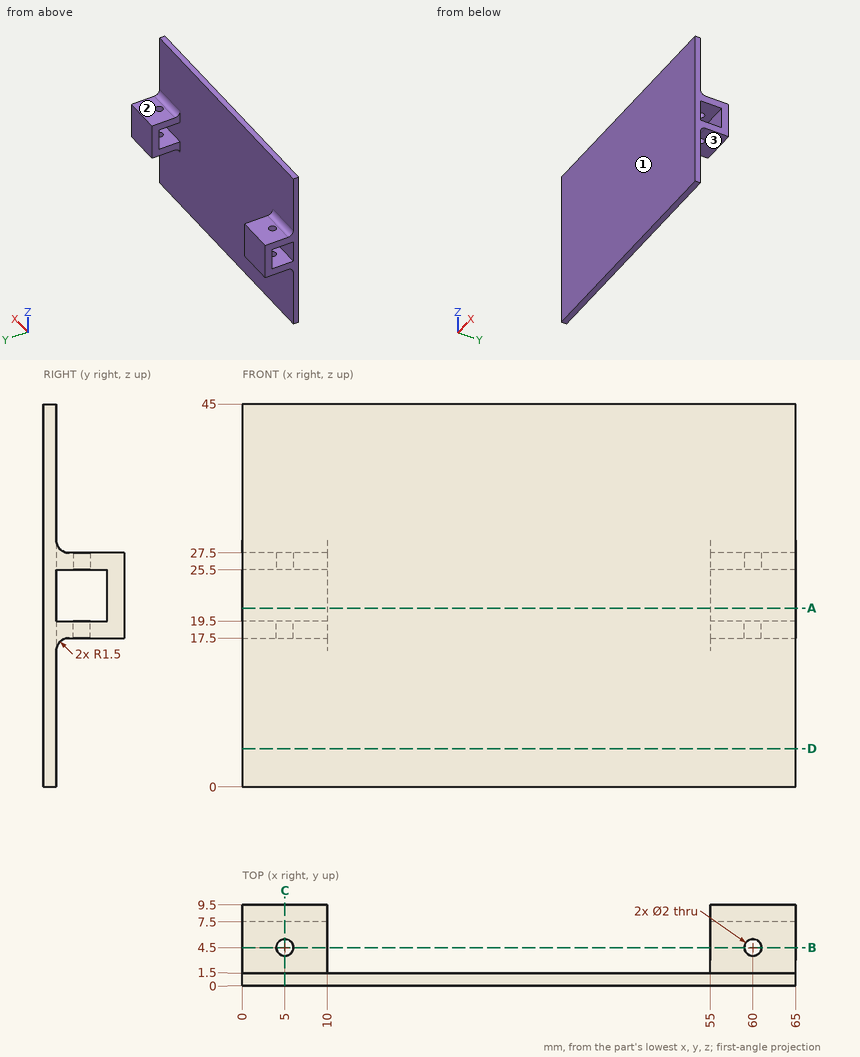
Study the drawing (mm; zero at the part's minimum x, y, z) and answer. A direction names the side the tool comes from. Coordinates: 2 decimals unless noted, no trailing zeros. Write each loop counter-clockwise with the first axis right and the second up, starting at its lowest first coordinate (ties: lowest second). Pieces come first, ordered by that corner, then holes. Notation, with made-up numbers: (-10.75, 46.5) - (43.25, 46.5) arc R31 ccw to (43.25, 78.5) - close; hole circle Ø10 at (86.25, 10.5). An arc over 180 degrees is marked (long way). Answer as a JSON object with one key per item and string values. Group by question number.
1. A cutting plane is placed at C-C (x = 5). Determine the outline of the cut face in (y, z), plus the area to 3 significant figures.
2. A cutting plane is placed at A-A (z = 21). Determine the outline of the cut face in (x, y).
3. Each of these flat-tipped pins is pushed along its axis until it touches: P1, Ø2.5, axis at x = 5, y = 4.5, coming from the -Z side; P2, Ø5, axis at x = 30, y = 3.5, coming from the +Z side; P3, Ø3, axis at x = 58.5, y = 4.5, coming from the +Z side; P4, Ø3, axis at x = 7, y = 4, coming from the -Z side. Where does it stop, or does it pass through?
4. A cutting plane is placed at D-D (z = 4.5). Determine the outline of the cut face in (x, y), plus the area to 3 significant figures.
5. Which of the six approach directions +Z, -Z, +X, -X, +Y, -Y give full straight-line access (tool end or side, diameter ignored) to the marked faces 1, 2 and 3?
6. A cutting plane is placed at B-B (y = 4.5). Give the number of separate pieces and of enclosed holes in the cut face, plus the area to 3 significant figures.
7. Consider L1, parallel to X at y = 4.5, z = 18.2; L2, parallel to Y at x = 60, z = 26.1; L3, parallel to Z at x = 62, y = 3.5. Determine where each line is inside the solid, lowest interval first. Write a range as [from, to].
Worked out:
{
 "1": {"outline": "(0, 0) - (1.5, 0) - (1.5, 16) arc R1.5 cw to (3, 17.5) - (3.5, 17.5) - (3.5, 19.5) - (1.5, 19.5) - (1.5, 25.5) - (3.5, 25.5) - (3.5, 27.5) - (3, 27.5) arc R1.5 cw to (1.5, 29) - (1.5, 45) - (0, 45) - close; (5.5, 17.5) - (9.5, 17.5) - (9.5, 27.5) - (5.5, 27.5) - (5.5, 25.5) - (7.5, 25.5) - (7.5, 19.5) - (5.5, 19.5) - close", "area": "104 mm²"},
 "2": {"outline": "(0, 0) - (65, 0) - (65, 1.5) - (0, 1.5) - close; (0, 7.5) - (10, 7.5) - (10, 9.5) - (0, 9.5) - close; (55, 7.5) - (65, 7.5) - (65, 9.5) - (55, 9.5) - close"},
 "3": {"P1": "stops at z = 17.5", "P2": "stops at z = 45", "P3": "stops at z = 27.5", "P4": "stops at z = 17.41"},
 "4": {"outline": "(0, 0) - (65, 0) - (65, 1.5) - (0, 1.5) - close", "area": "97.5 mm²"},
 "5": {"face 1": "+Z, -Z, +X, -X, -Y", "face 2": "+Z, +X, -X, +Y", "face 3": "-Z, +X, -X, +Y"},
 "6": {"separate pieces": "8", "enclosed holes": "0", "area": "64.0 mm²"},
 "7": {"L1": "x = [0, 4], [6, 10], [55, 59], [61, 65]", "L2": "y = [0, 3.5], [5.5, 9.5]", "L3": "z = [17.5, 19.5], [25.5, 27.5]"}
}
